```python
from build123d import *

# Parameters (mm, degrees)
ESBO_O1_W                = 138.5
ESBO_O1_H                = 68.5
ESBO_O1_R                = 1.65
ESBO_O1_R_2              = 32.5
ESBO_O1_R_3              = 5
RESSALTO_EXTRUS_O1_DEPTH = 2
ESBO_O2_R                = 4.25
ESBO_O2_R_2              = 1.65
RESSALTO_EXTRUS_O2_DEPTH = 6


with BuildPart() as part:
    # Esboço1 → Ressalto-extrusão1 (new body)
    with BuildSketch(Plane.XY):
        Rectangle(ESBO_O1_W, ESBO_O1_H)
        with Locations((-65, 30)):
            Circle(ESBO_O1_R, mode=Mode.SUBTRACT)
        with Locations((-65, -20)):
            Circle(ESBO_O1_R, mode=Mode.SUBTRACT)
        with Locations((65, -20)):
            Circle(ESBO_O1_R, mode=Mode.SUBTRACT)
        with Locations((65, 30)):
            Circle(ESBO_O1_R, mode=Mode.SUBTRACT)
        Circle(ESBO_O1_R_2, mode=Mode.SUBTRACT)
        with Locations((-31, 31)):
            Circle(ESBO_O1_R, mode=Mode.SUBTRACT)
        with Locations((-31, -31)):
            Circle(ESBO_O1_R, mode=Mode.SUBTRACT)
        with Locations((31, -31)):
            Circle(ESBO_O1_R, mode=Mode.SUBTRACT)
        with Locations((31, 31)):
            Circle(ESBO_O1_R, mode=Mode.SUBTRACT)
        with Locations((45, 0)):
            Circle(ESBO_O1_R_3, mode=Mode.SUBTRACT)
    extrude(amount=RESSALTO_EXTRUS_O1_DEPTH)

    # Esboço2 → Ressalto-extrusão2 (add)
    with BuildSketch(Plane(origin=(0, 0, 0), x_dir=(-1, 0, 0), z_dir=(0, 0, -1))):
        with Locations((65, 30)):
            Circle(ESBO_O2_R)
        with Locations((65, 30)):
            Circle(ESBO_O2_R_2, mode=Mode.SUBTRACT)
        with Locations((65, -20)):
            Circle(ESBO_O2_R)
        with Locations((65, -20)):
            Circle(ESBO_O2_R_2, mode=Mode.SUBTRACT)
        with Locations((-65, -20)):
            Circle(ESBO_O2_R)
        with Locations((-65, -20)):
            Circle(ESBO_O2_R_2, mode=Mode.SUBTRACT)
        with Locations((-65, 30)):
            Circle(ESBO_O2_R)
        with Locations((-65, 30)):
            Circle(ESBO_O2_R_2, mode=Mode.SUBTRACT)
    extrude(amount=RESSALTO_EXTRUS_O2_DEPTH)


solid = part.part
```
Model file for the job. Use its own axes, mm. A direction names the side the tool comes from. Give positions to 0.01 mm unless a question says otherwise; leave off trailing zeros. Loops run counter-clockwise (first coordinate to the right, second up) from the corner with the lowest first, then second, coordinate; pieces in that order, holes last. Notation, with made-up numbers: (42.25, -17.75) - (66.25, -17.75) arc R12 ccw to (66.25, -7.75) - close; hole circle Ø9 at (31.5, 28.5). An arc over 180 degrees is marked (long way). One line per item, written item: value. Start each with the question number.
1. Which spindle directions (+Z, -Z, +X, -X, +Y, -Y) get a long thin tool onto all of the face, cutting with end or side? Do faces 4 (the flat face through (-68.4, 33.2, 0)), 5 (the cylindrical face through (61.074, -21.628, -2.958)), 6 (the flat face through (-32, -7, 2)). Say none if no direction does.
2. Slice it at B-B (y = 0). List the corners of the cut face in (x, z), plus the area to 3 significant figures.
3. Pull direction Y, two halves, no side cores. Call faces 1 (the flat face through (-32, -7, 0)), 2 (the cylindrical face through (-31.215, 32.636, 0.986)), 3 (the flat face through (68.2, 33.4, 0)): pulls with the +Y half, pulls with the -Y half, needs draft (parallel to the pull), parting line crosses it, or undercut.
4. Slice it at D-D (x = 45). List the corners of the cut face in (y, z), plus the area to 3 significant figures.
5. Slice it at C-C (y = -26). List the corners of the cut face in (x, z), plus the area to 3 significant figures.
6. Probe L1, parallel to Y at x = -65, z = 1.5; L2, parallel to Y at x = -65, z = -2; L3, parallel to X at y = -2, z = 1. List the from-to ranges inside material, lowest first. Write a range as from..to.
7. Pin check, flat tips, straight feed: pin 1 (20.5 mm diameter, centred on x = -7.5, y = 12, fed in from -Z); pin 2 (4 mm diameter, centred on x = 31, y = -31, fed in from -Z); pin 3 (5.5 mm diameter, centred on x = 65, y = 30, fed in from -Z). Stop position of each tip, or through.
8. Slice it at A-A (z = -3.25). List the corners of the cut face in (x, y).
Solution:
1. face 4: -Z, -X, +Y
1. face 5: -Z
1. face 6: +Z, +X, -X, +Y, -Y
2. outline: (-69.25, 0) - (-32.5, 0) - (-32.5, 2) - (-69.25, 2) - close; (32.5, 0) - (40, 0) - (40, 2) - (32.5, 2) - close; (50, 0) - (69.25, 0) - (69.25, 2) - (50, 2) - close
2. area: 127 mm^2
3. face 1: undercut
3. face 2: undercut
3. face 3: needs draft
4. outline: (-34.25, 0) - (-5, 0) - (-5, 2) - (-34.25, 2) - close; (5, 0) - (34.25, 0) - (34.25, 2) - (5, 2) - close
4. area: 117 mm^2
5. outline: (-69.25, 0) - (-19.5, 0) - (-19.5, 2) - (-69.25, 2) - close; (19.5, 0) - (69.25, 0) - (69.25, 2) - (19.5, 2) - close
5. area: 199 mm^2
6. L1: y = -34.25..-21.65, -18.35..28.35, 31.65..34.25
6. L2: y = -24.25..-21.65, -18.35..-15.75, 25.75..28.35, 31.65..34.25
6. L3: x = -69.25..-32.44, 32.44..40.42, 49.58..69.25
7. pin 1: passes through
7. pin 2: stops at z = 0
7. pin 3: stops at z = -6
8. outline: circle Ø8.5 at (-65, -20); circle Ø8.5 at (-65, 30); circle Ø8.5 at (65, -20); circle Ø8.5 at (65, 30); hole circle Ø3.3 at (-65, -20); hole circle Ø3.3 at (-65, 30); hole circle Ø3.3 at (65, -20); hole circle Ø3.3 at (65, 30)
